For this review, take the finished solid that the model builds, in its own axes (mm). Give positions to 0.01 mm unless a question says otherwise; leave off trailing zeros. Loops run counter-clockwise (first coordinate to the right, second up) from the corner with the lowest first, then second, coordinate; pieces in that order, holes last. Notation, with made-up numbers: (4.5, -2.5) - (58.5, -2.5) arc R11 cw to (58.5, 9.5) - close; hole circle Ø3 at (32.25, 25.5). An arc over 180 degrees is marked (long way). Use CSV: the item, a comma, the result in double quotes. Start each with the question number.
1. Take a section at A-A on z = 1.9. State how many separate pieces and enclosed holes the cut face has, plus the area to 3 significant figures.
2. Wall thickness on line 1 (Y direction, x = 165.1, z = 2.2); line 2 (Y direction, x = -441.96, z = 1.7); line 3 (Y direction, x = 274.5, z = 1.55): over which ranges is each line inside the solid? List them lowest first.
3. Take a section at B-B on x = 228. Give the boundary of the cut face in (y, z) (3 decimals), plus the area to 3 significant figures.
```python
from build123d import *

# Parameters (mm, degrees)
BOSS_EXTRUDE1_DEPTH            = 3.175
F_1_4_CLEARANCE_HOLE1_D        = 6.7564
F_5_16_0_3125_DIAMETER_HOLE1_D = 7.9375
F_1_4_0_25_DIAMETER_HOLE1_D    = 6.35


with BuildPart() as part:
    # Sketch2 → Boss-Extrude1 (new body)
    with BuildSketch(Plane.XY):
        Polygon((-482.6, 901.7), (-215.9, 901.7), (-215.9, 990.6), (215.9, 990.6), (215.9, 901.7), (482.6, 901.7), (482.6, 0), (-482.6, 0), align=None)
    extrude(amount=BOSS_EXTRUDE1_DEPTH)

    # 1/4 Clearance Hole1 (through all)
    with Locations(Plane.XY.offset(3.175)):
        with Locations((-441.96, 311.50918615), (105.907561142, 362.110143283), (289.91643105, 312.805115191), (-289.91643105, 312.805115191), (-105.907561142, 362.110143283), (441.96, 311.50918615)):
            Hole(F_1_4_CLEARANCE_HOLE1_D / 2)

    # 5/16 (0.3125) Diameter Hole1 (through all)
    with Locations(Plane.XY.offset(3.175)):
        with Locations((-165.1, 922.02), (-165.1, 965.2), (165.1, 965.2), (165.1, 922.02), (-165.1, 210.82), (-165.1, 254), (165.1, 254), (165.1, 210.82), (-444.5, 177.8), (444.5, 177.8), (-444.5, 889), (444.5, 889)):
            Hole(F_5_16_0_3125_DIAMETER_HOLE1_D / 2)

    # 1/4 (0.25) Diameter Hole1 (through all)
    with Locations(Plane.XY.offset(3.175)):
        with Locations((0, 889), (12.7, 889)):
            Hole(F_1_4_0_25_DIAMETER_HOLE1_D / 2)


solid = part.part
```
Check result:
1,separate pieces,"1"
1,enclosed holes,"20"
1,area,"908,000 mm²"
2,line 1,"y = 0 to 206.85, 214.79 to 250.03, 257.97 to 918.05, 925.99 to 961.23, 969.17 to 990.6"
2,line 2,"y = 0 to 174.75, 180.85 to 308.13, 314.89 to 885.95, 892.05 to 901.7"
2,line 3,"y = 0 to 901.7"
3,outline,"(0, 0) - (901.7, 0) - (901.7, 3.175) - (0, 3.175) - close"
3,area,"2,860 mm²"
